```python
from build123d import *


with BuildPart() as f2:
    # F2: sweep along a path in F1
    with BuildLine(Plane.YZ) as f2_path:
        Line((0, 0), (-106.027229, 0))
        ThreePointArc((-106.027229, 0), (-150.92851, -18.598719), (-169.527229, -63.5))
        Line((-169.527229, -63.5), (-169.527229, -149.079217))
        ThreePointArc((-169.527229, -149.079217), (-165.771549, -170.593545), (-154.948762, -189.562962))
        Line((-154.948762, -189.562962), (-88.474994, -269.891465))
    # F0 (on Front) → F2 (sweep)
    with BuildSketch(Plane.XZ):
        Polygon((-35.452579, 21.786269), (-40.473978, -9.663541), (-21.786269, -35.452579), (9.663541, -40.473978), (35.452579, -21.786269), (40.473978, 9.663541), (21.786269, 35.452579), (-9.663541, 40.473978), align=None)
    sweep(path=f2_path.line)


solid = f2.part
```
The listing builds one solid part. Answer for the finished solid, in the listing's coordinates (mm). A direction names the side the tool comes from. Give positions to 0.01 mm unless a question says otherwise; leave off trailing zeros. Loops run counter-clockwise (first coordinate to the right, second up) from the corner with the lowest first, then second, coordinate; pieces in that order, holes last. Notation, with made-up numbers: (46, -11.75) - (89, -11.75) arc R31 ccw to (89, 18.25) - close; hole circle Ø3 at (51, 46.25). An arc over 180 degrees is marked (long way). Return JSON: item names as keys, results as strings. Group by question number.
1. Find section A-A (z = -85.5). Write down the section's boundary in (x, y), then the cut area to 3 significant figures.
2. Given pin 1 Ø5 at (x, z) = (-14.5, -262) entering from +Y; pin 2 Ø2 at (x, z) = (-17, 5) entering from +Y; pin 3 Ø4 at (x, z) = (6, -19) entering from -Y; pin 4 Ø1 at (x, y) = (-17.5, -167) entering from +Z, each flat-ended and moving along its own axis, determine where each tip first touches the part or whether it passes through.
3. Determine the mould class of faces 4 (the flat face through (31.261, -191.905, -106.889)), 5 (the conical face through (19.87, -127.3, -41.75)), 6 (the flat face through (-37.93, -126.09, -234.29)) for opening direction Z: pulls with the +Z half, pulls with the -Z half, needs draft (parallel to the pull), parting line crosses it, or undercut.
4. Find section C-C (y = -54). Write down the section's boundary in (x, z).
5. Find section D-D (x = -26.5). Write down the section's boundary in (y, z), then the cut area to 3 significant figures.
6. Which of the six approach directions +Z, -Z, +X, -X, +Y, -Y give full straight-line access (tool end or side, diameter ignored) to faces 1 (the flat face through (22.38, -138.27, -106.89)), 2 (the flat face through (-31.26, -147.15, -106.89)), 3 (the flat face through (6.28, -53.76, 37.93))?
7. Find section B-B (y = -101.5). Write down the section's boundary in (x, z).
8. Straight lines are drawn through the part: line 1 (Z direction, x = -15.5, y = -95.5); line 2 (Z direction, x = 10, y = -77); line 3 (Y direction, x = -17.5, z = -180). For each, find the intervals that lie inside material, in ascending order. Write a range as [from, to].
Verdict:
{
 "1": {"outline": "(-40.47, -159.86) - (-35.45, -191.31) - (-9.66, -210) - (21.79, -204.98) - (40.47, -179.19) - (35.45, -147.74) - (9.66, -129.05) - (-21.79, -134.07) - close", "area": "4,900 mm^2"},
 "2": {"pin 1": "stops at y = -75.92", "pin 2": "stops at y = 0", "pin 3": "stops at y = -198.24", "pin 4": "stops at z = 14.2"},
 "3": {"face 4": "needs draft", "face 5": "undercut", "face 6": "pulls with the -Z half"},
 "4": {"outline": "(-40.47, -9.66) - (-21.79, -35.45) - (9.66, -40.47) - (35.45, -21.79) - (40.47, 9.66) - (21.79, 35.45) - (-9.66, 40.47) - (-35.45, 21.79) - close"},
 "5": {"outline": "(-197.8, -149.08) arc R91.77 ccw to (-176.73, -207.59) - (-110.26, -287.92) - (-66.17, -251.44) - (-132.65, -171.11) arc R34.55 cw to (-140.58, -149.08) - (-140.58, -63.5) arc R34.55 cw to (-106.03, -28.95) - (0, -28.95) - (0, 28.27) - (-106.03, 28.27) arc R91.77 ccw to (-197.8, -63.5) - close", "area": "25,100 mm^2"},
 "6": {"face 1": "+X, +Y", "face 2": "-X, +Y", "face 3": "+Z, +X, +Y, -Y"},
 "7": {"outline": "(-40.47, -238.99) - (-36.23, -280.67) - (35.23, -280.67) - (40.47, -269.31) - (35.45, -219.98) - (9.66, -190.67) - (-21.79, -198.54) - close; (-40.47, -9.66) - (-21.79, -35.45) - (9.66, -40.47) - (35.45, -21.79) - (40.47, 9.66) - (21.79, 35.45) - (-9.66, 40.47) - (-35.45, 21.79) - close"},
 "8": {"line 1": "z = [-275.7, -204.22], [-36.46, 36.24]", "line 2": "z = [-260.4, -220.66], [-40.23, 37.33]", "line 3": "y = [-199.33, -115.96]"}
}
